Check sheet for the modelled part. Datum: model origin and axes. Units: mm. Face numbers are marked on the shaded views. Round coordinates to 2 decimals unless told otherwise and drop trailing zeros. Order: outer loops, then holes, each group sorted by start corner. A loop starts at its lowest first (then second) coordinate and runs counter-clockwise, first axis right, second up.
Q1. Scan lines: probe 1 along Y at (x, z) = (0, 18.5); probe 2 along Y at (x, z) = (-37, 4.75); probe 3 along Y at (x, z) = (-58.5, 15). Record each from-to range of solid material in increasing order.
Q2. Cross-section at D-D on y = 56.5. Record the cut outline in (x, z).
Q3. Cross-section at B-B on y = 0. Record the cut outline in (x, z), then the cut area to 3 significant figures.
Q4. Cross-section at C-C on z = 17. Give the number of separate pieces and of enclosed holes in the cut face, then the cut area to 3 significant figures.
Q5. Depth check by flat-ended pin: P1, Ø24.5, axis at x = 0, y = 56.5, coming from the -Z side; P2, Ø12, axis at y = 45, z = 5.5, coming from the +X side; P3, Ø3, axis at y = 41, z = 20, coming from the +X side; P4, Ø2, axis at x = -71.5, z = 15.5, coming from the -Y side. Enter the tip coordinate at first touch or a pass-through.
Q6. Mould release check, pull along Y, two halves, no side actions. Record for the marked faces 1, 2, 3 and 4: +Y half, -Y half, draft (parallel to the pull), parting line (faces both ways), or undercut.
Q7. Cross-section at A-A on x = 0. Record the cut outline in (y, z), then the cut area to 4 significant figures.
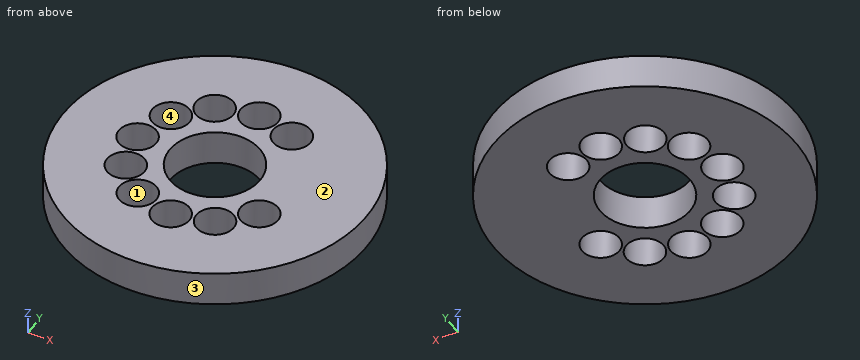
from build123d import *

# Parameters (mm, degrees)
F0_R     = 109
F0_R_2   = 75
F0_R_3   = 13.5
F0_R_4   = 37.5
F0_R_5   = 32.5
F1_DEPTH = 25


with BuildPart() as f1:
    # F0 (on Top) → F1 (new body)
    with BuildSketch(Plane.XY):
        Circle(F0_R)
        Circle(F0_R_2, mode=Mode.SUBTRACT)
        Circle(F0_R_2)
        with Locations((-28.408734, -48.838446)):
            Circle(F0_R_3, mode=Mode.SUBTRACT)
        with Locations((-48.848327, -28.391741)):
            Circle(F0_R_3, mode=Mode.SUBTRACT)
        with Locations((0, -56.5)):
            Circle(F0_R_3, mode=Mode.SUBTRACT)
        with Locations((28.099003, -49.017303)):
            Circle(F0_R_3, mode=Mode.SUBTRACT)
        with Locations((48.722864, -28.606512)):
            Circle(F0_R_3, mode=Mode.SUBTRACT)
        with Locations((-56.5, 0)):
            Circle(F0_R_3, mode=Mode.SUBTRACT)
        with Locations((-48.624626, 28.773177)):
            Circle(F0_R_3, mode=Mode.SUBTRACT)
        with Locations((-28.228625, 48.94277)):
            Circle(F0_R_3, mode=Mode.SUBTRACT)
        Circle(F0_R_4, mode=Mode.SUBTRACT)
        with Locations((28.012047, 49.067048)):
            Circle(F0_R_3, mode=Mode.SUBTRACT)
        with Locations((0, 56.5)):
            Circle(F0_R_3, mode=Mode.SUBTRACT)
        Circle(F0_R_4)
        Circle(F0_R_5, mode=Mode.SUBTRACT)
    extrude(amount=F1_DEPTH)


solid = f1.part
Results found:
1. probe 1: y = -109 to -70, -43 to -32.5, 32.5 to 43, 70 to 109
1. probe 2: y = -102.53 to -59.25, -38.42 to -34.86, -21.92 to 21.91, 35.64 to 38.68, 59.2 to 102.53
1. probe 3: y = -91.97 to -37.83, -18.95 to -13.35, 13.35 to 19.57, 37.98 to 91.97
2. outline: (-93.21, 0) - (-39.42, 0) - (-39.42, 25) - (-93.21, 25) - close; (-17.04, 0) - (-13.5, 0) - (-13.5, 25) - (-17.04, 25) - close; (13.5, 0) - (16.74, 0) - (16.74, 25) - (13.5, 25) - close; (39.28, 0) - (93.21, 0) - (93.21, 25) - (39.28, 25) - close
3. outline: (-109, 0) - (-70, 0) - (-70, 25) - (-109, 25) - close; (-43, 0) - (-32.5, 0) - (-32.5, 25) - (-43, 25) - close; (32.5, 0) - (109, 0) - (109, 25) - (32.5, 25) - close
3. area: 3,150 mm2
4. separate pieces: 1
4. enclosed holes: 11
4. area: 28,300 mm2
5. P1: passes through
5. P2: stops at x = 101.78
5. P3: stops at x = 101.59
5. P4: stops at y = -83.13
6. face 1: undercut
6. face 2: draft
6. face 3: parting line
6. face 4: undercut
7. outline: (-109, 0) - (-70, 0) - (-70, 25) - (-109, 25) - close; (-43, 0) - (-32.5, 0) - (-32.5, 25) - (-43, 25) - close; (32.5, 0) - (43, 0) - (43, 25) - (32.5, 25) - close; (70, 0) - (109, 0) - (109, 25) - (70, 25) - close
7. area: 2,475 mm2
